Geometry check sheet. Reference: the model listing, model coordinates, mm. A direction names the side the tool comes from. Give positions to 0.01 mm unless a question says otherwise; leave off trailing zeros. Loops run counter-clockwise (first coordinate to the right, second up) from the corner with the lowest first, then second, coordinate; pieces in that order, holes last. Notation, with made-up numbers: (24, 58.5) -> (33, 58.5) arc R21 cw to (33, 79.5) -> close; hole circle Ø9 at (23.25, 80). An arc over 180 degrees is marked (long way). One line per question, with ' | ' between items.
from build123d import *

# Parameters (mm, degrees)
EXTRUDE1_DEPTH     = 2.54
SKETCH2_W          = 44.45
SKETCH2_H          = 27.305
EXTRUDE2_DEPTH     = 0.8382
FILLET1_R          = 0.4191
SKETCH3_R          = 2.2225
CUT_EXTRUDE1_DEPTH = 74.109188914


with BuildPart() as part:
    # Sketch1 → Extrude1 (new body)
    with BuildSketch(Plane(origin=(0, 0, 0), x_dir=(1, 0, 0), z_dir=(0, 1, 0))):
        with BuildLine():
            Line((-35.8775, -62.8269), (35.8775, -62.8269))
            ThreePointArc((35.8775, -62.8269), (36.883288686, -62.410288686), (37.2999, -61.4045))
            Line((37.2999, -61.4045), (37.2999, 61.4045))
            ThreePointArc((37.2999, 61.4045), (36.883288686, 62.410288686), (35.8775, 62.8269))
            Line((35.8775, 62.8269), (-35.8775, 62.8269))
            ThreePointArc((-35.8775, 62.8269), (-36.883288686, 62.410288686), (-37.2999, 61.4045))
            Line((-37.2999, 61.4045), (-37.2999, -61.4045))
            ThreePointArc((-37.2999, -61.4045), (-36.883288686, -62.410288686), (-35.8775, -62.8269))
        make_face()
    extrude(amount=EXTRUDE1_DEPTH)

    # Sketch2 → Extrude2 (cut)
    with BuildSketch(Plane(origin=(0, 2.54, 0), x_dir=(1, 0, 0), z_dir=(0, 1, 0))):
        with Locations((7.7089, 35.2044)):
            Rectangle(SKETCH2_W, SKETCH2_H)
        with Locations((-7.7089, -35.2044)):
            Rectangle(SKETCH2_W, SKETCH2_H)
    extrude(amount=-EXTRUDE2_DEPTH, mode=Mode.SUBTRACT)

    # Fillet1
    fillet1_edges = [part.edges().sort_by_distance(p)[0] for p in [
        (-14.5161, 1.7018, -35.2044),
        (-14.5161, 2.1209, -21.5519),
        (7.7089, 1.7018, -48.8569),
        (-14.5161, 2.1209, -48.8569),
        (29.9339, 1.7018, -35.2044),
        (29.9339, 2.1209, -48.8569),
        (7.7089, 1.7018, -21.5519),
        (29.9339, 2.1209, -21.5519),
        (-14.5161, 2.54, -35.2044),
        (7.7089, 2.54, -21.5519),
        (29.9339, 2.54, -35.2044),
        (7.7089, 2.54, -48.8569),
        (-29.9339, 1.7018, 35.2044),
        (-29.9339, 2.1209, 48.8569),
        (-7.7089, 1.7018, 21.5519),
        (-29.9339, 2.1209, 21.5519),
        (14.5161, 1.7018, 35.2044),
        (14.5161, 2.1209, 21.5519),
        (-7.7089, 1.7018, 48.8569),
        (14.5161, 2.1209, 48.8569),
        (-29.9339, 2.54, 35.2044),
        (-7.7089, 2.54, 48.8569),
        (14.5161, 2.54, 35.2044),
        (-7.7089, 2.54, 21.5519),
    ]]
    fillet(fillet1_edges, radius=FILLET1_R - 0.0001)  # a hair under: the kernel refuses the full size

    # Sketch3 → Cut-Extrude1 (cut, through all)
    with BuildSketch(Plane(origin=(0, 2.54, 0), x_dir=(1, 0, 0), z_dir=(0, 1, 0))):
        with Locations(Location((31.75, 57.15, 0), (0, 0, 270))):
            Circle(SKETCH3_R)
        with Locations(Location((-31.75, -57.15, 0), (0, 0, 270))):
            Circle(SKETCH3_R)
    extrude(amount=-CUT_EXTRUDE1_DEPTH, mode=Mode.SUBTRACT)


solid = part.part
Item 1: Release check for a two-part mould opening along Z. For faces 1 (the face through (1, 1, -62.827)), 2 (the face through (37.3, 1, 1)), 3 (the face through (-1, 1, 62.827)), 4 (the face through (29.78, 1.29, -56.12)) record: pulls with the +Z half, pulls with the -Z half, needs draft (parallel to the pull), parting line crosses it, or undercut.
Result:
face 1: pulls with the -Z half | face 2: needs draft | face 3: pulls with the +Z half | face 4: undercut
Item 2: Set-up check for faces 5 (the face through (7, 1.702, -35)), 6 (the face through (-33.72, 1.29, 58.18)): record each of +Z, -Z, +X, -X, +Y, -Y from which the full face is reachable in a straight line by a thin tool's end or side.
Result:
face 5: +Y | face 6: +Y, -Y
Item 3: Sectioned sample at A-A (z = 57.15). Record the cut outline in (x, y).
Result:
outline: (-37.3, 0) -> (-33.97, 0) -> (-33.97, 2.54) -> (-37.3, 2.54) -> close; (-29.53, 0) -> (37.3, 0) -> (37.3, 2.54) -> (-29.53, 2.54) -> close
Item 4: Scan lines: probe 1 along X at (y, z) = (1.25, -57.15); probe 2 along Z at (x, y) = (6.5, 2.35); probe 3 along Z at (x, y) = (4.5, 1.9). Record each from-to range of solid material in increasing order.
Result:
probe 1: -37.3 to 29.53, 33.97 to 37.3 | probe 2: -62.83 to -48.93, -21.48 to 21.48, 48.93 to 62.83 | probe 3: -62.83 to -48.79, -21.61 to 21.61, 48.79 to 62.83
Item 5: Sectioned sample at B-B (x = -31.75). Record the cut outline in (y, z).
Result:
outline: (0, -62.83) -> (2.54, -62.83) -> (2.54, 54.93) -> (0, 54.93) -> close; (0, 59.37) -> (2.54, 59.37) -> (2.54, 62.83) -> (0, 62.83) -> close
Item 6: Depth check by flat-ended pin: pin 1 Ø8 at (x, z) = (15, -41.5) entering from +Y; pin 2 Ø5 at (x, z) = (31.75, -57.15) entering from +Y. Enter the tip coordinate at first touch or a pass-through.
Result:
pin 1: y = 1.7 | pin 2: y = 2.54
